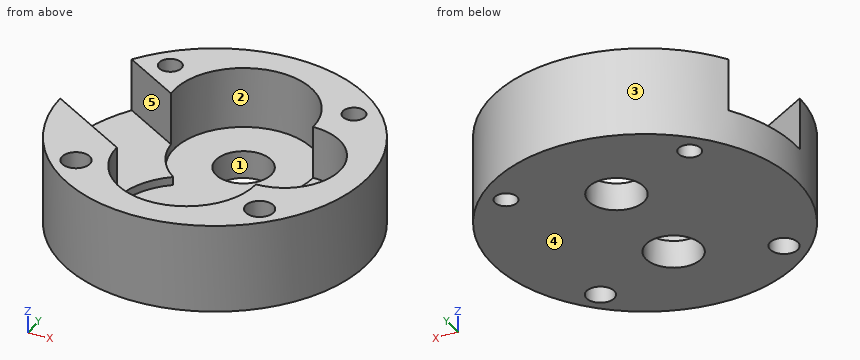
```python
from build123d import *

# Parameters (mm, degrees)
SKETCH1_R           = 55
BOSS_EXTRUDE1_DEPTH = 32
SKETCH1_19_R        = 10
CUT_EXTRUDE1_DEPTH  = 22
CUT_EXTRUDE2_DEPTH  = 19
SKETCH1_21_R        = 10
SKETCH1_21_R_2      = 4
SKETCH1_21_R_3      = 5
CUT_EXTRUDE3_DEPTH  = 85.107074613


with BuildPart() as part:
    # Sketch1 → Boss-Extrude1 (new body)
    with BuildSketch(Plane.XY):
        Circle(SKETCH1_R)
    extrude(amount=-BOSS_EXTRUDE1_DEPTH)

    # Sketch1<19> → Cut-Extrude1 (cut)
    # profile 1 of 3: a face of its own
    with BuildSketch(Plane.XY):
        with BuildLine():
            ThreePointArc((15, 0), (0, 45), (-15, 0))
            ThreePointArc((-15, 0), (0, -45), (15, 0))
        make_face()
        with Locations((0, -20)):
            Circle(SKETCH1_19_R, mode=Mode.SUBTRACT)
        with Locations((0, 20)):
            Circle(SKETCH1_19_R, mode=Mode.SUBTRACT)
    # profile 2 of 3: a face of its own
    with BuildSketch(Plane.XY):
        with Locations((0, -20)):
            Circle(SKETCH1_19_R)
    # profile 3 of 3: a face of its own
    with BuildSketch(Plane.XY):
        with Locations((0, 20)):
            Circle(SKETCH1_19_R)
    extrude(amount=-CUT_EXTRUDE1_DEPTH, mode=Mode.SUBTRACT)

    # Sketch1<20> → Cut-Extrude2 (cut)
    with BuildSketch(Plane.XY):
        with BuildLine():
            ThreePointArc((-45.668792135, 30.649003654), (-52.795976975, 15.41378653), (-54.985496966, -1.262981944))
            Line((-54.985496966, -1.262981944), (-25, -20))
            ThreePointArc((-25, -20), (-22.360679775, -8.819660113), (-15, 0))
            ThreePointArc((-15, 0), (-21.813646246, 7.786694246), (-24.890758601, 17.665447305))
            Line((-24.890758601, 17.665447305), (-45.668792135, 30.649003654))
        make_face()
        with BuildLine():
            ThreePointArc((15, 0), (22.360679775, -8.819660113), (25, -20))
            ThreePointArc((25, -20), (45, 0), (25, 20))
            ThreePointArc((25, 20), (22.360679775, 8.819660113), (15, 0))
        make_face()
    extrude(amount=-CUT_EXTRUDE2_DEPTH, mode=Mode.SUBTRACT)

    # Sketch1<21> → Cut-Extrude3 (cut, through all)
    with BuildSketch(Plane.XY):
        with Locations((0, 20)):
            Circle(SKETCH1_21_R)
        with Locations((0, -20)):
            Circle(SKETCH1_21_R)
        with Locations((-33, 33)):
            Circle(SKETCH1_21_R_2)
        with Locations((33, 33)):
            Circle(SKETCH1_21_R_2)
        with Locations((33, -33)):
            Circle(SKETCH1_21_R_3)
        with Locations((-33, -33)):
            Circle(SKETCH1_21_R_3)
    extrude(amount=-CUT_EXTRUDE3_DEPTH, mode=Mode.SUBTRACT)


solid = part.part
```
Can you work these out from the model? Positions are in its coordinate system, mm. Face numbers are marked on the shaded views. A direction names the side the tool comes from. Round coordinates to 2 decimals unless told otherwise and drop trailing zeros. Loops run counter-clockwise (first coordinate to the right, second up) from the corner with the lowest first, then second, coordinate; pieces in that order, holes last. Notation, with made-up numbers: M 44.5,4.5 L 98.5,4.5 A22 ccw 98.5,33.5 Z; hole C 75.5,58 d4. An arc over 180 degrees is marked long. Write item = value, one per line. Start each with the question number.
(1) Suppose I cut it at D-D on y = -33. Write out the boundary of the cut face in (x, z), plus the area to 3 significant figures.
(2) I need wall thicknesses on line 1 along Y through (x, z) = (0, -25.5); line 2 along Y through (x, z) = (0, -6.5); line 3 along Y through (x, z) = (36, -25). Which ranges of each line are inside material? Lowest first, please.
(3) Suppose I cut it at C-C on x = -33. Write out the boundary of the cut face in (y, z), plus the area to 3 significant figures.
(4) If we mould it in two halves opening along Y, with no side actions, what happens to the marked faces 3, 4 and 5? For each: released by +Y, released by -Y, zero draft, split by the parting line, or undercut.
(5) Which directions (+Z, -Z, +X, -X, +Y, -Y) give clear straight access to the entire face, cutting with the end or side of a thin tool? Please do the marked faces 1 and 2.
(6) Suppose I cut it at B-B on y = 26. Write out the boundary of the cut face in (x, z).
(7) I'm going to push flat-ended pins straight in: P1, Ø3, axis at x = -13.5, z = -14, coming from the -Y side; P2, Ø11.5, axis at x = 33, y = -33, coming from the -Z side; P3, Ø20, axis at x = -39.5, y = 7, coming from the +Z side; P4, Ø4, axis at x = 11.5, z = -8, coming from the +Y side. Where does each tip first touch, or does it pass through?
(8) Suppose I cut it at A-A on z = -11. Write out the boundary of the cut face in (x, y).
Answer block:
q1.outline = M -44,-32 L -38,-32 L -38,0 L -44,0 Z; M -28,-32 L 28,-32 L 28,0 L 21.35,0 L 21.35,-22 L -21.35,-22 L -21.35,0 L -28,0 Z; M 38,-32 L 44,-32 L 44,0 L 38,0 Z
q1.area = 1,240 mm²
q2.line_1 = -55 to -30, -10 to 10, 30 to 55
q2.line_2 = -55 to -45, 45 to 55
q2.line_3 = -41.58 to -37, -29 to 30.35, 35.65 to 41.58
q3.outline = M -44,-32 L -38,-32 L -38,0 L -44,0 Z; M -28,-32 L 29,-32 L 29,0 L 22.73,0 L 22.73,-19 L -15,-19 L -15,0 L -28,0 Z; M 37,-32 L 44,-32 L 44,0 L 37,0 Z
q3.area = 1,520 mm²
q4.face_3 = split by the parting line
q4.face_4 = zero draft
q4.face_5 = undercut
q5.face_1 = +Z, -Z
q5.face_2 = +Z
q6.outline = M -48.47,-32 L -8,-32 L -8,-22 L -24.27,-22 L -24.27,0 L -38.23,0 L -38.23,-19 L -48.47,-19 Z; M 8,-32 L 48.47,-32 L 48.47,0 L 24.27,0 L 24.27,-22 L 8,-22 Z
q7.P1 = -53.67
q7.P2 = -32
q7.P3 = -19
q7.P4 = 54.17
q8.outline = M -54.99,-1.26 A55 ccw long -45.67,30.65 L -24.89,17.67 A25 cw long 25,20 A20 cw 25,-20 A25 cw -25,-20 Z; hole C -33,-33 d10; hole C -33,33 d8; hole C 33,-33 d10; hole C 33,33 d8
